from build123d import *

# Parameters (mm, degrees)
ESBO_O1_W                = 150
ESBO_O1_H                = 30
RESSALTO_EXTRUS_O1_DEPTH = 10
ESBO_O2_R                = 13
CORTE_EXTRUS_O1_DEPTH    = 8
CORTE_EXTRUS_O2_REACH    = 78.903
ESBO_O3_R                = 9
CORTE_EXTRUS_O3_REACH    = 83.394
ESBO_O4_W                = 65
ESBO_O4_H                = 10


with BuildPart() as part:
    # Esboço1 → Ressalto-extrusão1 (new body)
    with BuildSketch(Plane.XY):
        Rectangle(ESBO_O1_W, ESBO_O1_H)
    extrude(amount=RESSALTO_EXTRUS_O1_DEPTH)

    # Esboço2 → Corte-extrusão1 (cut)
    with BuildSketch(Plane.XY.offset(10)):
        with Locations((-60, 0)):
            Circle(ESBO_O2_R)
    extrude(amount=-CORTE_EXTRUS_O1_DEPTH, mode=Mode.SUBTRACT)

    # Esboço3 → Corte-extrusão2 (cut, up to next)
    with BuildSketch(Plane.XY.offset(2), mode=Mode.PRIVATE) as corte_extrus_o2_sk1:
        with Locations((-60, 0)):
            Circle(ESBO_O3_R)
    corte_extrus_o2_tool1 = extrude(corte_extrus_o2_sk1.sketch, amount=-CORTE_EXTRUS_O2_REACH, mode=Mode.PRIVATE) & part.part
    add(corte_extrus_o2_tool1.solids().sort_by_distance((-60, 0, 2))[0], mode=Mode.SUBTRACT)

    # Esboço4 → Corte-extrusão3 (cut, up to next)
    with BuildSketch(Plane.XZ.offset(15), mode=Mode.PRIVATE) as corte_extrus_o3_sk1:
        with Locations((42.5, 5)):
            Rectangle(ESBO_O4_W, ESBO_O4_H)
    corte_extrus_o3_tool1 = extrude(corte_extrus_o3_sk1.sketch, amount=-CORTE_EXTRUS_O3_REACH, mode=Mode.PRIVATE) & part.part
    add(corte_extrus_o3_tool1.solids().sort_by_distance((42.5, -15, 5))[0], mode=Mode.SUBTRACT)


solid = part.part
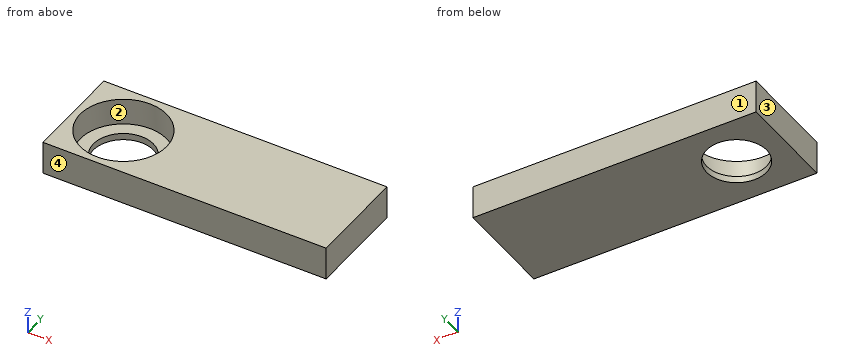
Design review of the part built by this model. Coordinates are the model's own, in mm. Face numbers are marked on the shaded views. Give positions to 0.01 mm unless a question says otherwise; leave off trailing zeros. Loops run counter-clockwise (first coordinate to the right, second up) from the corner with the lowest first, then second, coordinate; pieces in that order, holes last. Notation, with made-up numbers: M 16,89.25 L 63,89.25 A29 cw 63,115.25 Z; hole C 40,23.5 d4. An arc over 180 degrees is marked long. One line per question, with ' | ' between items. Start each with the question number.
1. Add section D-D (y = -12). Write out the cut boundary in (x, z), plus the area to 3 significant figures.
2. To check wall thickness, follow L1, parallel to Y at x = -60, z = 1; L2, parallel to Y at x = -60, z = 5.75; L3, parallel to Z at x = -50.5, y = 3. State the ranges of each line that lie inside material, in increasing order.
3. Add section B-B (x = -60). Write out the cut boundary in (y, z).
4. Add section A-A (y = 0). Write out the cut boundary in (x, z).
5. The part is to be moulded in two halves that separate along Y. For the marked faces 1, 2, 3 and 4, say which applies: released by +Y, released by -Y, zero draft, split by the parting line, or undercut.
6. Add section C-C (z = 4.75). Write out the cut boundary in (x, y), plus the area to 3 significant figures.
Worked out:
1) outline: M -75,0 L 10,0 L 10,10 L -55,10 L -55,2 L -65,2 L -65,10 L -75,10 Z | area: 770 mm²
2) L1: y = -15 to -9, 9 to 15 | L2: y = -15 to -13, 13 to 15 | L3: z = 0 to 2
3) outline: M -15,0 L -9,0 L -9,2 L -13,2 L -13,10 L -15,10 Z; M 9,0 L 15,0 L 15,10 L 13,10 L 13,2 L 9,2 Z
4) outline: M -75,0 L -69,0 L -69,2 L -73,2 L -73,10 L -75,10 Z; M -51,0 L 10,0 L 10,10 L -47,10 L -47,2 L -51,2 Z
5) face 1: released by +Y | face 2: undercut | face 3: zero draft | face 4: released by -Y
6) outline: M -75,-15 L 10,-15 L 10,15 L -75,15 Z; hole C -60,0 d26 | area: 2,020 mm²
